```python
from build123d import *

# Parameters (mm, degrees)
IZIM1_W                     = 68
IZIM1_H                     = 68
Y_KSEKLIK_EKSTR_ZYON1_DEPTH = 10
IZIM2_W                     = 40
IZIM2_H                     = 40
Y_KSEKLIK_EKSTR_ZYON2_DEPTH = 28
IZIM3_R                     = 3
KES_EKSTR_ZYON1_DEPTH       = 20
IZIM4_R                     = 3
KES_EKSTR_ZYON2_DEPTH       = 20
IZIM5_R                     = 3
KES_EKSTR_ZYON3_DEPTH       = 101.159872204


with BuildPart() as part:
    # Çizim1 → Yükseklik-Ekstrüzyon1 (new body)
    with BuildSketch(Plane.XY):
        with Locations((-34, -34)):
            Rectangle(IZIM1_W, IZIM1_H)
    extrude(amount=Y_KSEKLIK_EKSTR_ZYON1_DEPTH)

    # Çizim2 → Yükseklik-Ekstrüzyon2 (add)
    with BuildSketch(Plane.XY.offset(10)):
        with Locations((-48, -20)):
            Rectangle(IZIM2_W, IZIM2_H)
    extrude(amount=Y_KSEKLIK_EKSTR_ZYON2_DEPTH)

    # Çizim3 → Kes-Ekstrüzyon1 (cut)
    with BuildSketch(Plane.XZ.offset(40)):
        with Locations(Location((-42, 24, 0), (0, 0, 270))):
            Circle(IZIM3_R)
    extrude(amount=-KES_EKSTR_ZYON1_DEPTH, mode=Mode.SUBTRACT)

    # Çizim4 → Kes-Ekstrüzyon2 (cut)
    with BuildSketch(Plane(origin=(-28, 0, 0), x_dir=(0, 0, -1), z_dir=(1, 0, 0))):
        with Locations(Location((-24, -26, 0), (0, 0, 90))):
            Circle(IZIM4_R)
    extrude(amount=-KES_EKSTR_ZYON2_DEPTH, mode=Mode.SUBTRACT)

    # Çizim5 → Kes-Ekstrüzyon3 (cut, through all)
    with BuildSketch(Plane.XY.offset(10)):
        with Locations((-14, -54)):
            Circle(IZIM5_R)
        with Locations((-14, -16)):
            Circle(IZIM5_R)
        with Locations((-52, -54)):
            Circle(IZIM5_R)
    extrude(amount=-KES_EKSTR_ZYON3_DEPTH, mode=Mode.SUBTRACT)


solid = part.part
```
The model under review builds one solid part; all positions refer to its coordinate system, in mm. A direction names the side the tool comes from. Round coordinates to 2 decimals unless told otherwise and drop trailing zeros. Order: outer loops, then holes, each group sorted by start corner. A loop starts at its lowest first (then second) coordinate and runs counter-clockwise, first axis right, second up.
(1) Tool access review of faces 1 (the face through (-48, -26, 24)), 2 (the face through (-42, -20, 24)), 3 (the face through (-48, -40, 24)): name each direction out of +Z, -Z, +X, -X, +Y, -Y from which nothing blocks a thin tool from reaching the whole face with its end or side.
Working result:
face 1: +X
face 2: -Y
face 3: +Z, +X, -X, -Y
(2) Mouldability with a two-part tool opening along Y and no side actions: class faces 4 (the face through (-42, 0, 15)), 5 (the face through (-54.21, -51.97, 5.07)), 6 (the face through (-45.62, -23.14, 24.9)), 7 (the face through (-48, -20, 38)) as released by +Y, released by -Y, zero draft, split by the parting line, or undercut.
Working result:
face 4: released by +Y
face 5: undercut
face 6: undercut
face 7: zero draft
(3) Take a section at C-C, the plane y = -37. State the section outline as (x, z) points, plus the area to 3 significant figures.
Working result:
outline: (-68, 0) - (0, 0) - (0, 10) - (-28, 10) - (-28, 38) - (-68, 38) - close; hole circle Ø6 at (-42, 24)
area: 1,770 mm2
(4) Take a section at A-A, the plane z = 4.5. State the section outline as (x, y) points, plus the area to 3 significant figures.
Working result:
outline: (-68, -68) - (0, -68) - (0, 0) - (-68, 0) - close; hole circle Ø6 at (-52, -54); hole circle Ø6 at (-14, -54); hole circle Ø6 at (-14, -16)
area: 4,540 mm2
(5) For P1, Ø14, axis at y = -25.5, z = 26, coming from the +X side; P2, Ø5.5, axis at x = -14, y = -54, coming from the -Z side; P3, Ø1.8, axis at x = -42, z = 23, coming from the -Y side; P4, Ø10, axis at x = -41, y = -46, coming from the +Z side, all flat-tipped, find the tip position at first contact; note any pin that passes through.
Working result:
P1: stops at x = -28
P2: passes through
P3: stops at y = -20
P4: stops at z = 10
(6) Wall thickness on L1, parallel to Y at x = -14, z = 7.75; L2, parallel to Z at x = -37.75, y = -26; L3, parallel to X at y = -22.8, z = 24: over which ranges is each line inside the solid? List them lowest first.
Working result:
L1: y = -68 to -57, -51 to -19, -13 to 0
L2: z = 0 to 21, 27 to 38
L3: x = -68 to -45, -39 to -28
(7) Take a section at D-D, the plane z = 25. State the section outline as (x, y) points, plus the area to 3 significant figures.
Working result:
outline: (-68, -40) - (-44.83, -40) - (-44.83, -28.83) - (-48, -28.83) - (-48, -23.17) - (-44.83, -23.17) - (-44.83, -20) - (-39.17, -20) - (-39.17, -23.17) - (-28, -23.17) - (-28, 0) - (-68, 0) - close; (-39.17, -40) - (-28, -40) - (-28, -28.83) - (-39.17, -28.83) - close
area: 1,410 mm2
(8) Take a section at B-B, the plane y = -54. State the section outline as (x, z) points, plus the area to 3 significant figures.
Working result:
outline: (-68, 0) - (-55, 0) - (-55, 10) - (-68, 10) - close; (-49, 0) - (-17, 0) - (-17, 10) - (-49, 10) - close; (-11, 0) - (0, 0) - (0, 10) - (-11, 10) - close
area: 560 mm2
